from build123d import *

# Parameters (mm, degrees)
SKETCH1_W           = 30
SKETCH1_H           = 75
BOSS_EXTRUDE1_DEPTH = 12
CUT_EXTRUDE1_DEPTH  = 12
LPATTERN1_COUNT     = 3
LPATTERN1_PITCH     = 20


with BuildPart() as part:
    # Sketch1 → Boss-Extrude1 (new body)
    with BuildSketch(Plane(origin=(0, 0, 0), x_dir=(1, 0, 0), z_dir=(0, 1, 0))):
        with Locations((15, 37.5)):
            Rectangle(SKETCH1_W, SKETCH1_H)
    extrude(amount=BOSS_EXTRUDE1_DEPTH)

    # Sketch3 → Cut-Extrude1 (cut)
    with BuildSketch(Plane(origin=(0, 0, 0), x_dir=(1, 0, 0), z_dir=(0, 1, 0))):
        Polygon((0, 5), (22.5, 12.5), (0, 20), align=None)
    cut_extrude1 = extrude(amount=CUT_EXTRUDE1_DEPTH, mode=Mode.SUBTRACT)

    # LPattern1: Cut-Extrude1 ×3
    with Locations(*[(0, 0, -i * LPATTERN1_PITCH) for i in range(1, LPATTERN1_COUNT)]):
        add(cut_extrude1, mode=Mode.SUBTRACT)


solid = part.part
The listing builds one solid part. Answer for the finished solid, in the listing's coordinates (mm). A direction names the side the tool comes from. Give positions to 0.01 mm unless a question says otherwise; leave off trailing zeros. Loops run counter-clockwise (first coordinate to the right, second up) from the corner with the lowest first, then second, coordinate; pieces in that order, holes last. Notation, with made-up numbers: (-3.75, 55) - (17.25, 55) arc R35 cw to (17.25, 89) - close; hole circle Ø6 at (23, 26.5). An arc over 180 degrees is marked (long way). Answer as a JSON object with one key per item and string values.
1. For a pull along Z with two mould halves and no side action, classify faces 1 (the flat face through (15, 6, -75)), 2 (the flat face through (11.1, 5.9, -48.7)), 3 (the flat face through (0, 6, -2)) as pulls with the +Z half, pulls with the -Z half, needs draft (parallel to the pull), parting line crosses it, or undercut.
Determined:
{"face 1": "pulls with the -Z half", "face 2": "undercut", "face 3": "needs draft"}
2. A cutting plane is placed at B-B (y = 11). Write down the section's boundary in (x, z).
Determined:
{"outline": "(0, -75) - (30, -75) - (30, 0) - (0, 0) - (0, -5) - (22.5, -12.5) - (0, -20) - (0, -25) - (22.5, -32.5) - (0, -40) - (0, -45) - (22.5, -52.5) - (0, -60) - close"}
3. For faces 4 (the flat face through (11.4, 5.9, -36.2)), 5 (the flat face through (0, 6, -67)), determine the directions among +Z, -Z, +X, -X, +Y, -Y from which every point of the face is accessible in a straight line to the end or side of a thin tool.
Determined:
{"face 4": "-X, +Y, -Y", "face 5": "+Z, -Z, -X, +Y, -Y"}
4. A cutting plane is placed at C-C (x = 17). Write down the section's boundary in (y, z).
Determined:
{"outline": "(0, -75) - (12, -75) - (12, -54.33) - (0, -54.33) - close; (0, -50.67) - (12, -50.67) - (12, -34.33) - (0, -34.33) - close; (0, -30.67) - (12, -30.67) - (12, -14.33) - (0, -14.33) - close; (0, -10.67) - (12, -10.67) - (12, 0) - (0, 0) - close"}
5. A cutting plane is placed at D-D (z = -37.5). Write down the section's boundary in (x, y).
Determined:
{"outline": "(7.5, 0) - (30, 0) - (30, 12) - (7.5, 12) - close"}
6. Find the intervals of material crossed by L1, parallel to Z at x = 20.25, y = 3.25; L2, parallel to Z at x = 19.25, y = 3.5, in increasing order. Write a range as [from, to].
Determined:
{"L1": "[-75, -53.25], [-51.75, -33.25], [-31.75, -13.25], [-11.75, 0]", "L2": "[-75, -53.58], [-51.42, -33.58], [-31.42, -13.58], [-11.42, 0]"}
7. A cutting plane is placed at A-A (x = 2.75). Write down the section's boundary in (y, z).
Determined:
{"outline": "(0, -75) - (12, -75) - (12, -59.08) - (0, -59.08) - close; (0, -45.92) - (12, -45.92) - (12, -39.08) - (0, -39.08) - close; (0, -25.92) - (12, -25.92) - (12, -19.08) - (0, -19.08) - close; (0, -5.92) - (12, -5.92) - (12, 0) - (0, 0) - close"}
